```python
from build123d import *

# Parameters (mm, degrees)
BOSS_EXTRUDE1_DEPTH             = 6.35
BOSS_EXTRUDE6_DEPTH             = 5.08
FILLET14_R                      = 5.08
FILLET16_R                      = 1.905
FILLET17_R                      = 1.27
FILLET18_R                      = 0.762
F_4_40_TAPPED_HOLE2_D           = 2.2606
F_4_40_TAPPED_HOLE2_CSINK_D     = 4.1148
F_4_40_TAPPED_HOLE2_CSINK_ANGLE = 100


with BuildPart() as part:
    # Sketch1 → Boss-Extrude1 (new body)
    with BuildSketch(Plane(origin=(0, 0, 0), x_dir=(1, 0, 0), z_dir=(0, 1, 0))):
        with BuildLine():
            Line((-32.253592819, 37.099138511), (-40.254592819, 23.241))
            Line((-40.254592819, 23.241), (-52.351555238, 2.288446473))
            Line((-52.351555238, 2.288446473), (-61.152528051, 7.369690496))
            ThreePointArc((-61.152528051, 7.369690496), (7.45083255, -61.142694734), (57.593043611, 21.839994338))
            Line((57.593043611, 21.839994338), (45.017092819, 14.992108029))
            Line((45.017092819, 14.992108029), (35.492092819, 31.489891971))
            Line((35.492092819, 31.489891971), (47.93867456, 38.67592929))
            ThreePointArc((47.93867456, 38.67592929), (32.807858132, 52.130494624), (14.131882123, 59.951930183))
            ThreePointArc((14.131882123, 59.951930183), (4.380709214, 43.075056101), (-13.323695155, 51.227866526))
            ThreePointArc((-13.323695155, 51.227866526), (-20.56358212, 48.774524619), (-27.374593602, 45.30393787))
            Line((-27.374593602, 45.30393787), (-32.253592819, 37.099138511))
        make_face()
    extrude(amount=BOSS_EXTRUDE1_DEPTH)

    # Sketch11 → Boss-Extrude6 (add)
    with BuildSketch(Plane(origin=(0, 6.35, 0), x_dir=(1, 0, 0), z_dir=(0, 1, 0))):
        with BuildLine():
            Line((-51.642474306, -2.520350645), (-59.315900126, 1.909903818))
            ThreePointArc((-59.315900126, 1.909903818), (8.075233998, -58.794679489), (56.604538416, 17.831151702))
            Line((56.604538416, 17.831151702), (55.18302034, 17.057103335))
            ThreePointArc((55.18302034, 17.057103335), (15.941309212, -55.515629949), (-55.825680829, -14.819037351))
            Line((-55.825680829, -14.819037351), (-24.769862567, 38.840617327))
            Line((-24.769862567, 38.840617327), (-26.96822824, 40.112933469))
            Line((-26.96822824, 40.112933469), (-51.642474306, -2.520350645))
        make_face()
        with BuildLine():
            Line((42.534833803, 39.075547615), (43.942550941, 39.888293484))
            ThreePointArc((43.942550941, 39.888293484), (31.224480147, 50.468362167), (16.080037332, 57.1266675))
            Line((16.080037332, 57.1266675), (15.64988416, 55.598485895))
            ThreePointArc((15.64988416, 55.598485895), (30.242639161, 49.208670827), (42.534833803, 39.075547615))
        make_face()
    extrude(amount=BOSS_EXTRUDE6_DEPTH)

    # Fillet14
    fillet14_edges = [part.edges().sort_by_distance(p)[0] for p in [
        (47.93867456, 3.175, -38.67592929),
        (57.593043611, 3.175, -21.839994338),
        (-61.152528051, 3.175, -7.369690496),
        (-27.374593602, 3.175, -45.30393787),
    ]]
    fillet(fillet14_edges, radius=FILLET14_R)

    # Fillet16
    fillet16_edges = [part.edges().sort_by_distance(p)[0] for p in [
        (45.017092819, 3.175, -14.992108029),
        (35.492092819, 3.175, -31.489891971),
        (-13.323695155, 3.175, -51.227866526),
        (14.131882123, 3.175, -59.951930183),
        (-32.253592819, 3.175, -37.099138511),
        (-52.351555238, 3.175, -2.288446473),
    ]]
    fillet(fillet16_edges, radius=FILLET16_R)

    # Fillet17
    fillet17_edges = [part.edges().sort_by_distance(p)[0] for p in [
        (-24.769862567, 8.89, -38.840617327),
        (-59.315900126, 8.89, -1.909903818),
        (55.18302034, 8.89, -17.057103335),
        (-55.825680829, 8.89, 14.819037351),
        (15.64988416, 8.89, -55.598485895),
        (42.534833803, 8.89, -39.075547615),
    ]]
    fillet(fillet17_edges, radius=FILLET17_R)

    # Fillet18
    # the kernel refuses this fillet: 0.762 mm, written as the material it takes off along each edge
    with BuildSketch(Plane(origin=(56.604538416, 6.35, -17.831151702), x_dir=(0.2914560828028139, 0, 0.9565842105101043), z_dir=(0, 1, 0))) as fillet18_piece_1:
        with BuildLine():
            CenterArc((1.111341465, -0.761966165), FILLET18_R, 89.460057438, 150.909144636)
            Line((0.734601677, -1.424318889), (0.696927698, -1.490554162))
            ThreePointArc((0.696927698, -1.490554162), (0.043911241, -0.591644128), (-0.074637174, -0.015353572))
            Line((-0.074637174, -0.015353572), (-0.000718081, 0.076196616))
            ThreePointArc((-0.000718081, 0.076196616), (0.559261138, 0.078835195), (1.119240357, 0.076196616))
            Line((1.119240357, 0.076196616), (1.118522276, 0))
        make_face()
    extrude(amount=9.086497787, mode=Mode.SUBTRACT)
    with BuildSketch(Plane(origin=(43.942550941, 6.35, -39.888293484), x_dir=(-0.9654520894435082, 0, 0.2605806266574016), z_dir=(0, 1, 0))) as fillet18_piece_2:
        with BuildLine():
            CenterArc((1.196678226, -0.641298996), FILLET18_R, 57.309434955, 150.909144636)
            Line((0.525241797, -1.001600428), (0.458098154, -1.037630571))
            ThreePointArc((0.458098154, -1.037630571), (0.192751008, -0.537440161), (-0.067818044, -0.034744107))
            Line((-0.067818044, -0.034744107), (-0.019587713, 0.073639402))
            ThreePointArc((-0.019587713, 0.073639402), (0.576256944, 0.232131105), (1.649391505, 0.0641299))
            Line((1.649391505, 0.0641299), (1.608235753, 0))
        make_face()
    extrude(amount=9.100589381, mode=Mode.SUBTRACT)
    with BuildSketch(Plane(origin=(-26.96822824, 6.35, -40.112933469), x_dir=(-0.5009118669957486, 0, 0.8654982966492963), z_dir=(0, 1, 0))) as fillet18_piece_3:
        with BuildLine():
            CenterArc((FILLET18_R, FILLET18_R), FILLET18_R, 180, 90)
            Line((0, FILLET18_R), (0, 0))
            Line((0, 0), (FILLET18_R, 0))
        make_face()
    extrude(amount=6.985, mode=Mode.SUBTRACT)
    with BuildSketch(Plane(origin=(16.080037332, 6.35, -57.1266675), x_dir=(0.960208894047144, 0, 0.2792827953755126), z_dir=(0, 1, 0))) as fillet18_piece_4:
        with BuildLine():
            CenterArc((1.021997529, -0.761971386), FILLET18_R, 89.503466107, 150.909144636)
            Line((0.645759664, -1.424609348), (0.608135877, -1.490873144))
            ThreePointArc((0.608135877, -1.490873144), (-0.073326676, -0.331878972), (-0.076197139, -0.000660352))
            Line((-0.076197139, -0.000660352), (-0.000660352, 0.076197139))
            ThreePointArc((-0.000660352, 0.076197139), (0.514300527, 0.078428517), (1.029261406, 0.076197139))
            Line((1.029261406, 0.076197139), (1.028601054, 0))
        make_face()
    extrude(amount=8.990336733, mode=Mode.SUBTRACT)
    with BuildSketch(Plane(origin=(-49.992695912, 11.43, 3.472850645), x_dir=(0, -1, 0), z_dir=(-0.8660254037844384, 0, -0.5000000000000006))) as fillet18_piece_5_section:
        with BuildLine():
            CenterArc((FILLET18_R, FILLET18_R), FILLET18_R, 180, 90)
            Line((0, FILLET18_R), (0, 0))
            Line((0, 0), (FILLET18_R, 0))
        make_face()
    fillet18_piece_5 = extrude(amount=8.600562568, mode=Mode.PRIVATE)
    fillet18_piece_5 = split(fillet18_piece_5, bisect_by=Plane(origin=(-51.641469253, 11.43, 2.518614067), z_dir=(-0.8654982966492973, 0, -0.5009118669957471)), keep=Keep.TOP, mode=Mode.PRIVATE)
    add(fillet18_piece_5, mode=Mode.SUBTRACT)
    with BuildSketch(Plane(origin=(-58.076001583, 11.43, 0.272421623), x_dir=(0.49999999999999845, 0, -0.8660254037844397), z_dir=(0.8660254037844397, 0, 0.49999999999999845))) as fillet18_piece_6:
        with BuildLine():
            CenterArc((1.27 - FILLET18_R, -FILLET18_R), FILLET18_R, 0, 90)
            Line((1.27 - FILLET18_R, 0), (1.27, 0))
            Line((1.27, 0), (1.27, -FILLET18_R))
        make_face()
    revolve(axis=Axis((-58.076001583, 11.43, 0.272421623), (0, 1, 0)), revolution_arc=120.268759804, mode=Mode.SUBTRACT)
    with BuildSketch(Plane(origin=(-26.013991134, 11.43, -41.761707724), x_dir=(0, -1, 0), z_dir=(-0.5009118669957471, 0, 0.8654982966492973))) as fillet18_piece_7_section:
        with BuildLine():
            CenterArc((FILLET18_R, FILLET18_R), FILLET18_R, 180, 90)
            Line((0, FILLET18_R), (0, 0))
            Line((0, 0), (FILLET18_R, 0))
        make_face()
    fillet18_piece_7 = extrude(amount=53.068657444, mode=Mode.PRIVATE)
    fillet18_piece_7 = split(fillet18_piece_7, bisect_by=Plane(origin=(-51.595805666, 11.43, 2.547294796), z_dir=(0.5000000000000006, 0, -0.8660254037844384)), keep=Keep.TOP, mode=Mode.PRIVATE)
    add(fillet18_piece_7, mode=Mode.SUBTRACT)
    with BuildSketch(Plane(origin=(0, 11.43, 0), x_dir=(0.761629515590845, 0, -0.6480127166814359), z_dir=(0.6480127166814359, 0, 0.761629515590845))) as fillet18_piece_8:
        with BuildLine():
            CenterArc((59.346640514 - FILLET18_R, -FILLET18_R), FILLET18_R, 0, 90)
            Line((59.346640514 - FILLET18_R, 0), (59.346640514, 0))
            Line((59.346640514, 0), (59.346640514, -FILLET18_R))
        make_face()
    revolve(axis=Axis((0, 11.43, 0), (0, 1, 0)), revolution_arc=35.726455219, mode=Mode.SUBTRACT)
    with BuildSketch(Plane(origin=(0, 11.43, 0), x_dir=(-0.9999889984830188, 0, 0.004690726268822115), z_dir=(-0.004690726268822115, 0, -0.9999889984830188))) as fillet18_piece_9:
        with BuildLine():
            CenterArc((59.346640514 - FILLET18_R, -FILLET18_R), FILLET18_R, 0, 90)
            Line((59.346640514 - FILLET18_R, 0), (59.346640514, 0))
            Line((59.346640514, 0), (59.346640514, -FILLET18_R))
        make_face()
    revolve(axis=Axis((0, 11.43, 0), (0, 1, 0)), revolution_arc=199.059052139, mode=Mode.SUBTRACT)
    with BuildSketch(Plane(origin=(-49.992695912, 11.43, 3.472850645), x_dir=(0, -1, 0), z_dir=(-0.8660254037844384, 0, -0.5000000000000006))) as fillet18_piece_10a_section:
        with BuildLine():
            CenterArc((FILLET18_R, FILLET18_R), FILLET18_R, 180, 90)
            Line((0, FILLET18_R), (0, 0))
            Line((0, 0), (FILLET18_R, 0))
        make_face()
    fillet18_piece_10a = extrude(amount=8.600562568, mode=Mode.PRIVATE)
    fillet18_piece_10a = split(fillet18_piece_10a, bisect_by=Plane(origin=(-51.641469253, 11.43, 2.518614067), z_dir=(0.8654982966492973, 0, 0.5009118669957471)), keep=Keep.TOP, mode=Mode.PRIVATE)
    with BuildSketch(Plane(origin=(-26.013991134, 11.43, -41.761707724), x_dir=(0, -1, 0), z_dir=(-0.5009118669957471, 0, 0.8654982966492973))) as fillet18_piece_10b_section:
        with BuildLine():
            CenterArc((FILLET18_R, FILLET18_R), FILLET18_R, 180, 90)
            Line((0, FILLET18_R), (0, 0))
            Line((0, 0), (FILLET18_R, 0))
        make_face()
    fillet18_piece_10b = extrude(amount=53.068657444, mode=Mode.PRIVATE)
    fillet18_piece_10b = split(fillet18_piece_10b, bisect_by=Plane(origin=(-51.595805666, 11.43, 2.547294796), z_dir=(-0.5000000000000006, 0, 0.8660254037844384)), keep=Keep.TOP, mode=Mode.PRIVATE)
    fillet18_piece_10 = fillet18_piece_10a & fillet18_piece_10b
    add(fillet18_piece_10, mode=Mode.SUBTRACT)

    # #4-40 Tapped Hole2 (through all)
    with Locations(Plane(origin=(0, 6.35, 0), x_dir=(1, 0, 0), z_dir=(0, 1, 0))):
        with Locations((-22.830825604, 35.196661052), (-50.276937356, -13.438454396), (50.307612814, -13.438454396), (25.237025094, 33.505861406)):
            CounterSinkHole(F_4_40_TAPPED_HOLE2_D / 2, F_4_40_TAPPED_HOLE2_CSINK_D / 2, counter_sink_angle=F_4_40_TAPPED_HOLE2_CSINK_ANGLE)


solid = part.part
```
CAD build for the part. Positions are in the model's coordinates, mm. A direction names the side the tool comes from. Give positions to 0.01 mm unless a question says otherwise; leave off trailing zeros. Loops run counter-clockwise (first coordinate to the right, second up) from the corner with the lowest first, then second, coordinate; pieces in that order, holes last. Notation, with made-up numbers: M 11,45 L 25,45 A15 ccw 25,53 Z; hole C 15.25,-6.5 d4. An arc over 180 degrees is marked long. Use one line per item in the form item = value.
Item 1: Flat gauge pins, fed straight in: pin 1 (5 mm diameter, centred on x = -10, y = 4, fed in from -Z); pin 2 (1.8 mm diameter, centred on x = 50.31, z = 13.44, fed in from -Y); pin 3 (1.5 mm diameter, centred on x = 31.5, z = -45.5, fed in from +Y); pin 4 (3 mm diameter, centred on x = 11.5, z = 24.5, fed in from -Y). Where does each tip first touch, or does it go through?
Determined:
pin_1 = -49.58
pin_2 = through
pin_3 = 6.35
pin_4 = 0
Item 2: Slice it at B-B (x = 0). List the corners of the cut face in (y, z) (3 decimals).
Determined:
outline = M 0,-42.396 L 6.35,-42.396 L 6.35,57.759 L 11.43,57.759 L 11.43,58.585 A0.762 ccw 10.668,59.347 L 6.35,59.347 L 6.35,61.595 L 0,61.595 Z
Item 3: Two-plate mould, pull along Z, no slides. Class faces 4 (the face through (31.37, 8.48, -50.38)), 5 (the face through (-1, 6.35, 0)), 6 (the face through (30, 11.43, -50)): pulls with the +Z half, pulls with the -Z half, needs draft (parallel to the pull), parting line crosses it, or undercut.
Determined:
face_4 = pulls with the -Z half
face_5 = undercut
face_6 = needs draft
Item 4: Which spindle directions (+Z, -Z, +X, -X, +Y, -Y) get a long thin tool onto all of the face, cutting with end or side? Do faces 1 (the face through (40.32, 3.13, -23.13)), 2 (the face through (16.932, 8.854, 55.222)), 3 (the face through (49.467, 3.131, -17.415)). Say none if no direction does.
Determined:
face_1 = +Y, -Y
face_2 = +Y
face_3 = -Z, +Y, -Y
Item 5: Drill centre lines: probe 1 along X at (y, z) = (2.5, 13.5); probe 2 along Y at (x, z) = (46, 24.5); probe 3 along Z at (x, y) = (-43.5, 9.5). Where is each one in solid material? Low to high. Write a range as from..to.
Determined:
probe_1 = -60.1..-51.41, -49.15..49.18, 51.44..60.1
probe_2 = 0..6.35
probe_3 = -11.55..-6.48, 38..40.37
